Geometry check sheet. Reference: the model listing, model coordinates, mm. Round coordinates to 2 decimals unless told otherwise and drop trailing zeros. Loops run counter-clockwise (first coordinate to the right, second up) from the corner with the lowest first, then second, coordinate; pieces in that order, holes last. Notation, with made-up numbers: M -39.75,-30 L -31.75,-30 A16 cw -31.75,-12 Z; hole C 70.25,85.25 d6. An arc over 180 degrees is marked long. Write item = value, one per line.
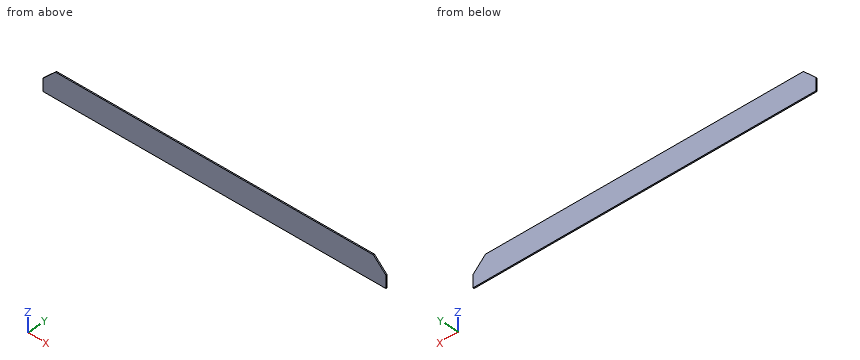
from build123d import *

# Parameters (mm, degrees)
F0_W     = 895
F0_H     = 3
F1_DEPTH = 65
F3_DEPTH = 3.001


with BuildPart() as f1:
    # F0 (on Top) → F1 (new body)
    with BuildSketch(Plane.XY):
        with Locations((447.5, 1.5)):
            Rectangle(F0_W, F0_H)
    extrude(amount=F1_DEPTH)

    # F2 (on face) → F3 (cut, through all)
    with BuildSketch(Plane.XZ):
        Polygon((895, 65), (862.5, 65), (895, 32.5), align=None)
        Polygon((0, 65), (0, 32.5), (32.5, 65), align=None)
    extrude(amount=-F3_DEPTH, mode=Mode.SUBTRACT)


solid = f1.part
(1) Material ranges on line 1 along X through (y, z) = (0.3, 36); line 2 along X through (y, z) = (1.6, 34.5), recorded low to high. Write a range as from..to.
Result set:
line_1 = 3.5..891.5
line_2 = 2..893
(2) Sectioned sample at A-A on y = 0.55. Record the cut outline in (x, z), then the cut area to 3 significant figures.
Result set:
outline = M 0,0 L 895,0 L 895,32.5 L 862.5,65 L 32.5,65 L 0,32.5 Z
area = 57,100 mm2
(3) Sectioned sample at B-B on z = 51. Record the cut outline in (x, y).
Result set:
outline = M 18.5,0 L 876.5,0 L 876.5,3 L 18.5,3 Z
